Verification items for the finished model (mm, model axes). A direction names the side the tool comes from. Round coordinates to 2 decimals unless told otherwise and drop trailing zeros. Order: outer loops, then holes, each group sorted by start corner. A loop starts at its lowest first (then second) coordinate and runs counter-clockwise, first axis right, second up. Notation, with made-up numbers: M -23,7.25 L -4,7.25 A25 cw -4,27.25 Z; hole C -17.5,0.5 d10. An arc over 180 degrees is marked long. Use one line per item in the form item = value. Start each with the question number.
Item 1: Release check for a two-part mould opening along Y. For faces 4 (the flat face through (0, -197, 35)), 5 (the cylindrical face through (25.52, -248.54, 6.76)), 6 (the flat face through (15, -30, -5)), 7 (the flat face through (0, 0, 16)) record: +Y half, -Y half, draft (parallel to the pull), parting line (faces both ways), or undercut.
Item 2: Cross-section at A-A on z = 0. Count the separate pieces of the cut face and the enclosed holes in it, then the cut area to 3 significant figures.
Item 3: Cross-section at C-C on y = -340. Enter the section's corners in (x, z), then the cut area to 3 significant figures.
Item 4: Cross-section at D-D on y = -275. Enter the section's corners in (x, z).
Item 5: Thickness scan on probe 1 along Z at (x, y) = (0, -309.5); probe 2 along Y at (x, z) = (27, -6); probe 3 along Z at (x, y) = (2, -201.5). Record the ranges inside material, lowest first. Write a range as [from, to].
Item 6: Tool access check on faces 1 (the cylindrical face through (-22.48, -217.59, 0.99)), 2 (the cylindrical face through (25.52, -178.54, 6.76)), 3 (the cylindrical face through (14.985, -14.79, 0.66)). Record the directions out of +Z, -Z, +X, -X, +Y, -Y that give a thin tool (end or side, any length) a straight path to the whole face; none if there is none.
Item 7: Go/stop test with flat-tipped pins: pin 1 Ø22.5 at (x, z) = (5, 3) entering from -Y; pin 2 Ø6 at (x, z) = (16.5, -9) entering from +Y. Record where each tip stops, or that it passes through.
Item 8: Cross-section at B-B on y = -156. Enter the section's corners in (x, z).
from build123d import *

# Parameters (mm, degrees)
F0_W     = 70
F0_H     = 70
F1_DEPTH = 400
F2_R     = 22.5
F3_DEPTH = 35
F4_R     = 22.5
F5_DEPTH = 370
F6_R     = 15
F7_DEPTH = 45


with BuildPart() as f1:
    # F0 (on Front) → F1 (new body)
    with BuildSketch(Plane.XZ):
        Rectangle(F0_W, F0_H)
    extrude(amount=F1_DEPTH)

    # F2 (on face) → F3 (cut)
    with BuildSketch(Plane.YZ.offset(35)):
        with Locations((-340, 0)):
            Circle(F2_R)
        with Locations((-270, 0)):
            Circle(F2_R)
        with Locations((-200, 0)):
            Circle(F2_R)
        with Locations((-130, 0)):
            Circle(F2_R)
        with Locations((-60, 0)):
            Circle(F2_R)
    extrude(amount=-F3_DEPTH, mode=Mode.SUBTRACT)

    # F4 (on face) → F5 (cut)
    with BuildSketch(Plane.XZ.offset(400)):
        Circle(F4_R)
    extrude(amount=-F5_DEPTH, mode=Mode.SUBTRACT)

    # F6 (on face) → F7 (cut)
    with BuildSketch(Plane(origin=(0, 0, 0), x_dir=(-1, 0, 0), z_dir=(0, 1, 0))):
        Circle(F6_R)
    extrude(amount=-F7_DEPTH, mode=Mode.SUBTRACT)


solid = f1.part
Output values:
q1.face_4 = draft
q1.face_5 = undercut
q1.face_6 = -Y half
q1.face_7 = +Y half
q2.separate_pieces = 7
q2.enclosed_holes = 0
q2.area = 7,640 mm2
q3.outline = M -35,-35 L 35,-35 L 35,-22.5 L 0,-22.5 A22.5 cw 0,22.5 L 35,22.5 L 35,35 L -35,35 Z
q3.area = 2,530 mm2
q4.outline = M -35,-35 L 35,-35 L 35,-21.94 L 5,-21.94 A22.5 cw long 5,21.94 L 35,21.94 L 35,35 L -35,35 Z
q5.probe_1 = [-35, -22.5], [22.5, 35]
q5.probe_2 = [-400, -361.69], [-318.31, -291.69], [-248.31, -221.69], [-178.31, -151.69], [-108.31, -81.69], [-38.31, 0]
q5.probe_3 = [-35, -22.45], [22.45, 35]
q6.face_1 = -Y
q6.face_2 = +X
q6.face_3 = +Y, -Y
q7.pin_1 = -30
q7.pin_2 = 0
q8.outline = M -35,-35 L 35,-35 L 35,35 L -35,35 Z; hole C 0,0 d45
